Can you work these out from the drawing? Everything is in mm from the part's minimum corner. Coordinates: 2 decimals unless noted, no trailing zeros. Order: outer loops, then holes, each group sorted by start corner. A loop starts at its lowest first (then second) coordinate and runs counter-clockwise, first axis right, second up. Notation, with made-up numbers: (36.25, -40) - (80.25, -40) arc R22 cw to (80.25, -11) - close; hole circle Ø1 at (-20.5, 71.25). An arc over 180 degrees is marked (long way). Use one line per item in the form item = value. Start each with the question number.
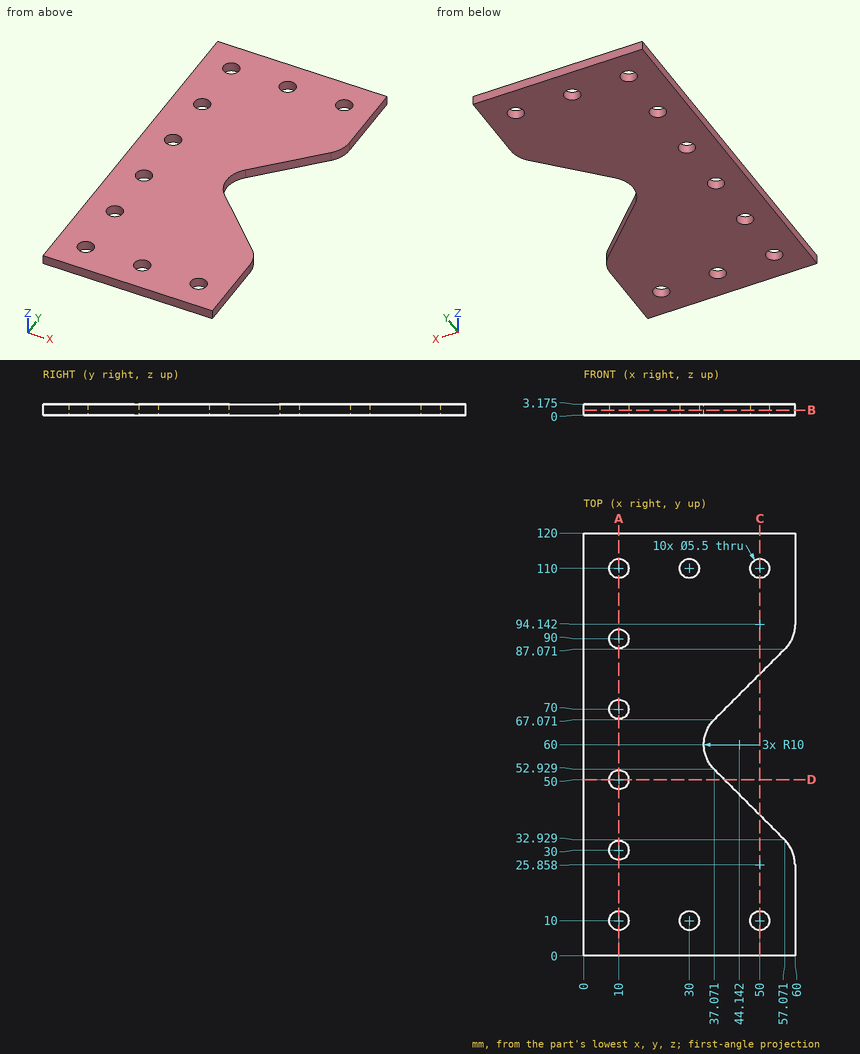
1) For pin 1 (1.5 mm diameter, centred on x = 27.5, y = 54.5, fed in from -Z); pin 2 (4.5 mm diameter, centred on x = 10, y = 90, fed in from -Z), each with a flat end and sliding along its axis, tell me the tip position at first contact or that it passes through.
2) Suppose I cut it at D-D, the plane y = 50. List the corners of the cut face in (x, z) for me (3 decimals).
3) I need wall thicknesses on probe 1 along Y at (x, z) = (30, 1.1); probe 2 along X at (y, z) = (9, 2.75); probe 3 along X at (y, z) = (28.5, 0.9) (1 decimal). Which ranges of each line are inside material? Lowest first, please. Write a range as [from, to].
4) Suppose I cut it at B-B, the plane z = 1.45. Give the number of separate pieces and of enclosed holes in the cut face, then the cut area to 3 significant figures.
5) Suppose I cut it at A-A, the plane x = 10. List the corners of the cut face in (y, z) for me (3 decimals), then the cut area to 3 significant figures.
6) Suppose I cut it at C-C, the plane x = 50. List the corners of the cut face in (y, z) for me (3 decimals).
From the geometry:
q1.pin_1 = 0
q1.pin_2 = through
q2.outline = (0, 0) - (7.25, 0) - (7.25, 3.175) - (0, 3.175) - close; (12.75, 0) - (40, 0) - (40, 3.175) - (12.75, 3.175) - close
q3.probe_1 = [0, 7.25], [12.75, 107.25], [112.75, 120]
q3.probe_2 = [0, 7.44], [12.56, 27.44], [32.56, 47.44], [52.56, 60]
q3.probe_3 = [0, 7.7], [12.3, 59.6]
q4.separate_pieces = 1
q4.enclosed_holes = 10
q4.area = 6,080 mm2
q5.outline = (0, 0) - (7.25, 0) - (7.25, 3.175) - (0, 3.175) - close; (12.75, 0) - (27.25, 0) - (27.25, 3.175) - (12.75, 3.175) - close; (32.75, 0) - (47.25, 0) - (47.25, 3.175) - (32.75, 3.175) - close; (52.75, 0) - (67.25, 0) - (67.25, 3.175) - (52.75, 3.175) - close; (72.75, 0) - (87.25, 0) - (87.25, 3.175) - (72.75, 3.175) - close; (92.75, 0) - (107.25, 0) - (107.25, 3.175) - (92.75, 3.175) - close; (112.75, 0) - (120, 0) - (120, 3.175) - (112.75, 3.175) - close
q5.area = 276 mm2
q6.outline = (0, 0) - (7.25, 0) - (7.25, 3.175) - (0, 3.175) - close; (12.75, 0) - (40, 0) - (40, 3.175) - (12.75, 3.175) - close; (80, 0) - (107.25, 0) - (107.25, 3.175) - (80, 3.175) - close; (112.75, 0) - (120, 0) - (120, 3.175) - (112.75, 3.175) - close
